from build123d import *

# Parameters (mm, degrees)
SKETCH_1_R      = 3.95
EXTRUDE_1_DEPTH = 120
EXTRUDE_2_DEPTH = 5.5
FILLET_1_R      = 0.3


with BuildPart() as part:
    # Эскиз1 → Бобышка-Вытянуть1 (new body)
    with BuildSketch(Plane.XY):
        Circle(SKETCH_1_R)
    extrude(amount=EXTRUDE_1_DEPTH)

    # Эскиз2 → Бобышка-Вытянуть2 (add)
    with BuildSketch(Plane(origin=(0, 0, 0), x_dir=(-1, 0, 0), z_dir=(0, 0, -1))):
        Polygon((-7.438440775, 0.373629267), (-4.042792825, -6.255064042), (3.395647951, -6.62869331), (7.438440775, -0.373629267), (4.042792825, 6.255064042), (-3.395647951, 6.62869331), align=None)
    extrude(amount=EXTRUDE_2_DEPTH)

    # Скругление1
    fillet_1_edges = [part.edges().sort_by_distance(p)[0] for p in [
        (-3.95, 0, 120),
        (-3.95, 0, 0),
        (5.417044363, 3.501161289, 0),
        (3.395647951, 6.62869331, -2.75),
        (5.7406168, -2.940717387, 0),
        (7.438440775, 0.373629267, -2.75),
        (0.323572437, -6.441878676, 0),
        (4.042792825, -6.255064042, -2.75),
        (-5.417044363, -3.501161289, 0),
        (-3.395647951, -6.62869331, -2.75),
        (-5.7406168, 2.940717387, 0),
        (-7.438440775, -0.373629267, -2.75),
        (-0.323572437, 6.441878676, 0),
        (-4.042792825, 6.255064042, -2.75),
        (5.417044363, 3.501161289, -5.5),
        (5.7406168, -2.940717387, -5.5),
        (0.323572437, -6.441878676, -5.5),
        (-5.417044363, -3.501161289, -5.5),
        (-5.7406168, 2.940717387, -5.5),
        (-0.323572437, 6.441878676, -5.5),
    ]]
    fillet(fillet_1_edges, radius=FILLET_1_R)


solid = part.part
Here's how the part is built. I have some questions about the finished solid (model axes, mm). A direction names the side the tool comes from. Coordinates: 2 decimals unless noted, no trailing zeros. Write each loop counter-clockwise with the first axis right and the second up, starting at its lowest first coordinate (ties: lowest second). Pieces come first, ordered by that corner, then holes.
1) Which directions (+Z, -Z, +X, -X, +Y, -Y) give clear straight access to the entire face, cutting with the end or side of a thin tool? Please do faces 1 (the face through (-3.135, -2.404, 59.164)), 2 (the face through (-5.638, 2.944, -5.414)).
Filled in:
face 1: +Z
face 2: -Z, -X, +Y
2) If we section it at A-A (z = 86): List the corners of the cut face in (x, y) for me.
Filled in:
outline: circle Ø7.9 at (0, 0)
3) I'm going to push flat-ended pins straight in: pin 1 (5 mm diameter, centred on y = 0, z = 66.5, fed in from +X); pin 2 (2 mm diameter, centred on x = -0.5, z = 77, fed in from +Y); pin 3 (5 mm diameter, centred on x = 4, z = 9, fed in from -Y). Where does each tip first touch, or does it pass through?
Filled in:
pin 1: stops at x = 3.95
pin 2: stops at y = 3.95
pin 3: stops at y = -3.65
4) If I drill on line 1 (Z direction, x = 3.5, y = 3.75); line 2 (X direction, y = 2.25, z = 29); line 3 (X direction, y = 0.5, z = 79), over which ranges is the centre line in solid material (lowest first)?
Filled in:
line 1: z = -5.5 to 0
line 2: x = -3.25 to 3.25
line 3: x = -3.92 to 3.92
